Check sheet for the modelled part. Datum: model origin and axes. Units: mm. Face numbers are marked on the shaded views. A direction names the side the tool comes from. Give positions to 0.01 mm unless a question says otherwise; leave off trailing zeros. Loops run counter-clockwise (first coordinate to the right, second up) from the corner with the lowest first, then second, coordinate; pieces in that order, holes last. Notation, with made-up numbers: (-37, -5) -> (5, -5) arc R19 cw to (5, 28) -> close; hole circle Ø3 at (23.5, 12.25). An arc over 180 degrees is marked (long way). Write each question's results on one line, items separated by ' | '. Start each with the question number.
1. Cross-section at D-D on x = 16.5. Record the boundary of the cut face in (y, z) (3 decimals).
2. Cross-section at A-A on z = -17. Record the boundary of the cut face in (x, y), and give its area (3 significant figures).
3. Tool access check on the marked faces 5, 6 and 7. Record the directions out of +Z, -Z, +X, -X, +Y, -Y that give a thin tool (end or side, any length) a straight path to the whole face; none if there is none.
4. Cross-section at C-C on y = -8. Record the boundary of the cut face in (x, z) (3 decimals).
5. Cross-section at B-B on z = 120.65. Record the boundary of the cut face in (x, y).
6. Material ranges on L1, parallel to Z at x = 14, y = 0 (3 decimals); L2, parallel to X at y = 0, z = 103; L3, parallel to X at y = 6, z = 65 (3 decimals), recorded low to high. Write a range as from..to.
7. Gauge pin test, flat ends, axial feed: pin 1 Ø2.5 at (y, z) = (0, 120.65) entering from +X; pin 2 Ø19 at (y, z) = (8, -35.5) entering from +X; pin 3 Ø11.5 at (y, z) = (4, -20.5) entering from -X; pin 4 Ø1.9 at (x, y) = (17, 1.5) entering from -Z. Record the tip position at first contact, or that the pin passes through.
8. Mould release check, pull along X, two halves, no side actions. Record for the marked faces 1, 2, 3 and 4: +X half, -X half, draft (parallel to the pull), parting line (faces both ways), or undercut.
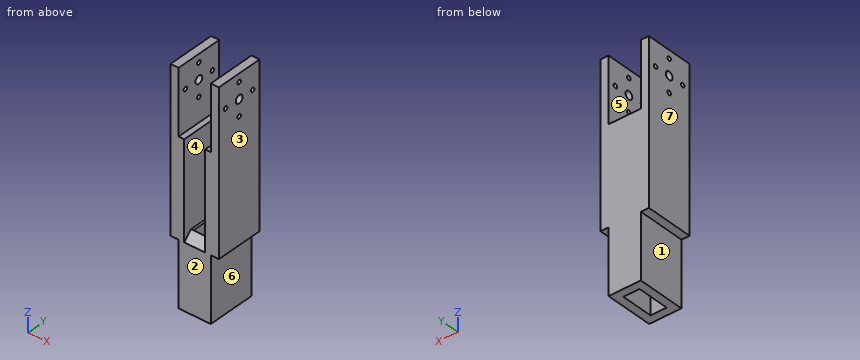
from build123d import *

# Parameters (mm, degrees)
F1_DEPTH = 6.35
F2_DEPTH = 76.2
F0_W     = 6.35
F0_H     = 38.1
F3_DEPTH = 127
F5_D     = 6.35
F6_SIZE  = 6.34999
F7_D     = 3.302
F8_DEPTH = 50.8


# Not quite as in the source:
# - a fillet or chamfer is up to 0.001 mm smaller than in the source, because OpenCascade refuses the exact size


with BuildPart() as f1:
    # F0 (on Top) → F1 (new body)
    with BuildSketch(Plane.XY):
        Polygon((-6.35, -12.7), (-6.35, 12.7), (-8.255, 12.7), (-8.255, -19.05), (8.255, -19.05), (8.255, 12.7), (6.35, 12.7), (6.35, -12.7), align=None)
    extrude(amount=F1_DEPTH)

    # F0 (on Top) → F2 (join)
    with BuildSketch(Plane.XY):
        Polygon((-8.255, -19.05), (-8.255, 12.7), (-8.255, 19.05), (-12.7, 19.05), (-12.7, -19.05), align=None)
        Polygon((8.255, 19.05), (8.255, 12.7), (8.255, -19.05), (12.7, -19.05), (12.7, 19.05), align=None)
        Polygon((-8.255, 12.7), (-6.35, 12.7), (6.35, 12.7), (8.255, 12.7), (8.255, 19.05), (-8.255, 19.05), align=None)
    extrude(amount=F2_DEPTH)

    # F0 (on Top) → F3 (join)
    with BuildSketch(Plane.XY):
        with Locations((-15.875, 0)):
            Rectangle(F0_W, F0_H)
        with Locations((15.875, 0)):
            Rectangle(F0_W, F0_H)
    extrude(amount=F3_DEPTH)

    # F5 (through all)
    with Locations(Plane.YZ.offset(19.05)):
        with Locations((0, 107.95)):
            Hole(F5_D / 2)

    # F6 (size 6.35 in the source; OpenCascade refuses exactly that, so slightly less here)
    f6_edges = [f1.edges().sort_by_distance(p)[0] for p in [
        (0, -19.05, 6.35),
    ]]
    chamfer(f6_edges, length=F6_SIZE)

    # F7 (through all)
    with Locations(Plane.YZ.offset(19.05)):
        with Locations((0, 120.65), (0, 95.25), (12.7, 107.95), (-12.7, 107.95)):
            Hole(F7_D / 2)

    # F0 (on Top) → F8 (join)
    with BuildSketch(Plane.XY):
        Polygon((-8.255, 12.7), (-6.35, 12.7), (6.35, 12.7), (8.255, 12.7), (8.255, 19.05), (-8.255, 19.05), align=None)
        Polygon((-8.255, -19.05), (-8.255, 12.7), (-8.255, 19.05), (-12.7, 19.05), (-12.7, -19.05), align=None)
        Polygon((-6.35, -12.7), (-6.35, 12.7), (-8.255, 12.7), (-8.255, -19.05), (8.255, -19.05), (8.255, 12.7), (6.35, 12.7), (6.35, -12.7), align=None)
        Polygon((8.255, 19.05), (8.255, 12.7), (8.255, -19.05), (12.7, -19.05), (12.7, 19.05), align=None)
    extrude(amount=-F8_DEPTH)


solid = f1.part
Geometry says:
1) outline: (-19.05, 0) -> (19.05, 0) -> (19.05, 127) -> (-19.05, 127) -> close; hole circle Ø3.302 at (-12.7, 107.95); hole circle Ø6.35 at (0, 107.95); hole circle Ø3.302 at (0, 95.25); hole circle Ø3.302 at (0, 120.65); hole circle Ø3.302 at (12.7, 107.95)
2) outline: (-12.7, -19.05) -> (12.7, -19.05) -> (12.7, 19.05) -> (-12.7, 19.05) -> close; hole (-6.35, -12.7) -> (6.35, -12.7) -> (6.35, 12.7) -> (-6.35, 12.7) -> close | area: 645 mm^2
3) face 5: +Z, +Y, -Y | face 6: -Z, +X, +Y, -Y | face 7: +Z, -Z, -X, +Y, -Y
4) outline: (-19.05, 0) -> (-12.7, 0) -> (-12.7, -50.8) -> (-6.35, -50.8) -> (-6.35, 6.35) -> (-8.255, 6.35) -> (-8.255, 76.2) -> (-12.7, 76.2) -> (-12.7, 127) -> (-19.05, 127) -> close; (6.35, -50.8) -> (12.7, -50.8) -> (12.7, 0) -> (19.05, 0) -> (19.05, 127) -> (12.7, 127) -> (12.7, 76.2) -> (8.255, 76.2) -> (8.255, 6.35) -> (6.35, 6.35) -> close
5) outline: (-19.05, -19.05) -> (-12.7, -19.05) -> (-12.7, -1.65) -> (-19.05, -1.65) -> close; (-19.05, 1.65) -> (-12.7, 1.65) -> (-12.7, 19.05) -> (-19.05, 19.05) -> close; (12.7, -19.05) -> (19.05, -19.05) -> (19.05, -1.65) -> (12.7, -1.65) -> close; (12.7, 1.65) -> (19.05, 1.65) -> (19.05, 19.05) -> (12.7, 19.05) -> close
6) L1: 0..93.599, 96.901..104.775, 111.125..118.999, 122.301..127 | L2: -19.05..-12.7, 12.7..19.05 | L3: -19.05..-8.255, 8.255..19.05
7) pin 1: through | pin 2: x = 12.7 | pin 3: x = -12.7 | pin 4: z = 0
8) face 1: -X half | face 2: draft | face 3: +X half | face 4: undercut
